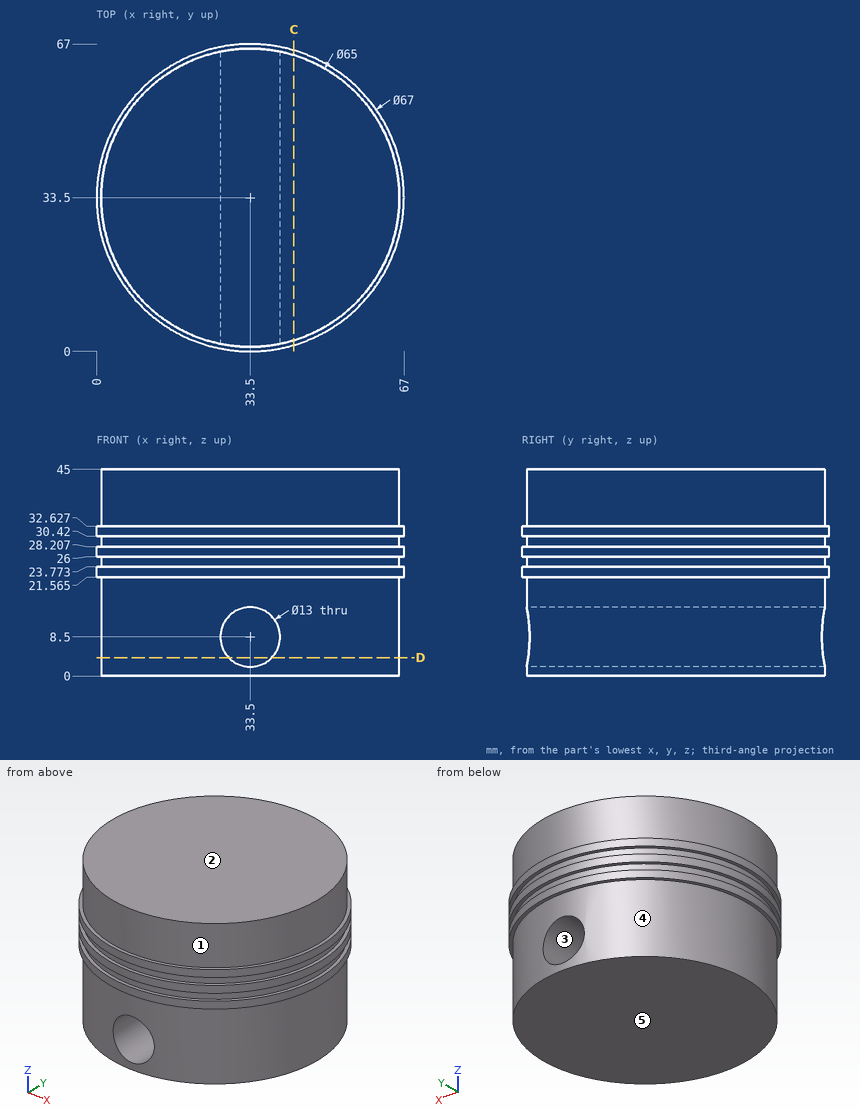
Input: dimensioned drawing with shaded views. Units: mm. Origin: part minimum x, y, z. A direction names the side the tool comes from. Coordinates: 2 decimals unless noted, no trailing zeros. Order: outer loops, then holes, each group sorted by start corner. A loop starts at its lowest first (then second) coordinate and runs counter-clockwise, first axis right, second up. Notation, with made-up numbers: (22.5, 75.25) - (77.5, 75.25) arc R23 cw to (77.5, 96.25) - close; hole circle Ø6 at (-11.75, -23). An arc over 180 degrees is marked (long way). Put each result on its own line as item: value.
1. Cut plane D-D on z = 4. Return the cut outline in (x, y), then the cut area to 3 significant figures.
Report:
outline: (28.81, 1.34) - (28.81, 65.66) arc R32.5 ccw to start; (38.19, 1.34) arc R32.5 ccw to (38.19, 65.66) - close
area: 2,710 mm2
2. Contact query for flat-ended pins moving along their axis: pin 1 Ø2 at (y, z) = (12, 9) entering from -X; pin 2 Ø4 at (y, z) = (50.5, 18.5) entering from +X; pin 3 Ø15 at (x, z) = (33.5, 8.5) entering from +Y. Output: stop coordinate, or through.
Report:
pin 1: stops at x = 8.28
pin 2: stops at x = 62.33
pin 3: stops at y = 66
3. Cut plane C-C on x = 43. Return the cut outline in (y, z) (1 decimal), then the cut area to 3 significant figures.
Report:
outline: (1.4, 21.6) - (2.4, 21.6) - (2.4, 0) - (64.6, 0) - (64.6, 21.6) - (65.6, 21.6) - (65.6, 23.8) - (64.6, 23.8) - (64.6, 26) - (65.6, 26) - (65.6, 28.2) - (64.6, 28.2) - (64.6, 30.4) - (65.6, 30.4) - (65.6, 32.6) - (64.6, 32.6) - (64.6, 45) - (2.4, 45) - (2.4, 32.6) - (1.4, 32.6) - (1.4, 30.4) - (2.4, 30.4) - (2.4, 28.2) - (1.4, 28.2) - (1.4, 26) - (2.4, 26) - (2.4, 23.8) - (1.4, 23.8) - close
area: 2,810 mm2
4. Line query: line 1 along Z through (x, y) = (33, 45); line 2 along X through (y, z) = (35, 8) (1 decimal); line 3 along X through (y, z) = (60, 14) (1 decimal). Output: solid intervals per line, ascending.
Report:
line 1: z = 0 to 2.02, 14.98 to 45
line 2: x = 1 to 27, 40 to 66
line 3: x = 14.7 to 30, 37 to 52.3
5. Draft query along X for the marked faces 3, 4 and 5. Return one class per face: pulls with the +X half, pulls with the -X half, needs draft (parallel to the pull), parting line crosses it, or undercut.
Report:
face 3: undercut
face 4: parting line crosses it
face 5: needs draft
6. Reachability of the marked faces 1 and 2 from +Z, -Z, +X, -X, +Y, -Y: full face, straight path, thin tool, end or side. Return the list, or none.
Report:
face 1: +Z
face 2: +Z, +X, -X, +Y, -Y
